Part print with two shaded views. Sizes in mm from the minimum x, y, z corner. A direction names the side the tool comes from. Round coordinates to 2 decimals unless told otherwise and drop trailing zeros. Write each loop counter-clockwise with the first axis right and the second up, starting at its lowest first coordinate (ties: lowest second). Pieces come first, ordered by that corner, then holes. Notation, with made-up numbers: (39, 58.5) -> (95, 58.5) arc R11 cw to (95, 76.5) -> close; hole circle Ø2 at (12.25, 12.5). An arc over 180 degrees is marked (long way). Return JSON: item names as keys, results as strings.
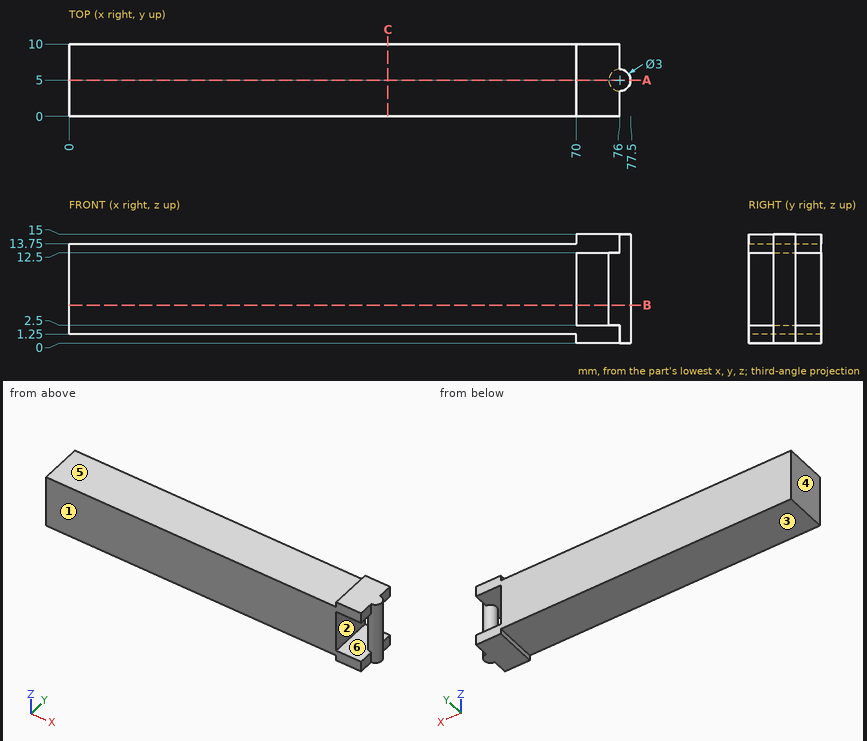
Q1. 3-axis set-ups, long thin cutter, end or side, ignore diameter. For the marked faces 1, 2 and 3: which of +Z, -Z, +X, -X, +Y, -Y reach the whole face in a straight line?
Verdict:
{"face 1": "+Z, -Z, +X, -X, -Y", "face 2": "+Y, -Y", "face 3": "-Z, -X, +Y, -Y"}
Q2. Two-plate mould, pull along X, no slides. Class the marked faces 4, 5 and 6: +X half, -X half, draft (parallel to the pull), parting line (faces both ways), or undercut.
Verdict:
{"face 4": "-X half", "face 5": "draft", "face 6": "undercut"}
Q3. Wall check: L1, parallel to X at y = 5, z = 4.25; L2, parallel to Z at x = 73, y = 3; L3, parallel to Z at x = 52.5, y = 5.5. Give the ranges that are in metal, low to high.
Verdict:
{"L1": "x = 0 to 70, 74.5 to 77.5", "L2": "z = 0 to 2.5, 12.5 to 15", "L3": "z = 1.25 to 13.75"}
Q4. Saw through at A-A on y = 5. List the corners of the cut face in (x, z), then the cut area to 4 significant figures.
Verdict:
{"outline": "(0, 1.25) -> (70, 1.25) -> (70, 0) -> (77.5, 0) -> (77.5, 15) -> (70, 15) -> (70, 13.75) -> (0, 13.75) -> close; hole (70, 2.5) -> (74.5, 2.5) -> (74.5, 12.5) -> (70, 12.5) -> close", "area": "942.5 mm²"}
Q5. Pin check, flat tips, straight feed: pin 1 Ø3 at (x, y) = (24, 5.5) entering from -Z; pin 2 Ø5 at (y, z) = (2, 6) entering from -X; pin 3 Ø1.2 at (y, z) = (1.5, 0.5) entering from +X; pin 4 Ø5 at (x, y) = (37, 3) entering from +Z. Stop position of each tip, or through.
Verdict:
{"pin 1": "stops at z = 1.25", "pin 2": "stops at x = 0", "pin 3": "stops at x = 76", "pin 4": "stops at z = 13.75"}
Q6. Saw through at C-C on x = 44. List the corners of the cut face in (y, z), then the cut area to 3 significant figures.
Verdict:
{"outline": "(0, 1.25) -> (10, 1.25) -> (10, 13.75) -> (0, 13.75) -> close", "area": "125 mm²"}
Q7. Saw through at B-B on z = 5.25. List the corners of the cut face in (x, y).
Verdict:
{"outline": "(0, 0) -> (70, 0) -> (70, 10) -> (0, 10) -> close; circle Ø3 at (76, 5)"}
